from build123d import *

# Parameters (mm, degrees)
F0_R     = 10.16
F1_DEPTH = 15.7734
F3_DEPTH = 40.2336
F4_R     = 3.302


with BuildPart() as f1:
    # F0 (on Top) → F1 (new body)
    with BuildSketch(Plane.XY):
        with BuildLine():
            ThreePointArc((8.651677, 27.233786), (23.06244, 16.871706), (28.575, 0))
            ThreePointArc((28.575, 0), (22.710053, -17.343129), (7.522744, -27.56699))
            Line((7.522744, -27.56699), (57.294815, -18.7585))
            ThreePointArc((57.294815, -18.7585), (34.935126, -0.621041), (56.065332, 18.934968))
            Line((56.065332, 18.934968), (8.651677, 27.233786))
        make_face()
        with BuildLine():
            Line((58.440289, 18.519279), (56.065332, 18.934968))
            ThreePointArc((56.065332, 18.934968), (34.935126, -0.621041), (57.294815, -18.7585))
            ThreePointArc((57.294815, -18.7585), (68.572003, -12.240507), (73.025, 0))
            ThreePointArc((73.025, 0), (68.941066, 11.786406), (58.440289, 18.519279))
        make_face()
        with Locations((53.975, 0)):
            Circle(F0_R, mode=Mode.SUBTRACT)
    extrude(amount=F1_DEPTH)

    # F2 (on Top) → F3 (join)
    with BuildSketch(Plane.XY):
        with BuildLine():
            ThreePointArc((7.522744, -27.56699), (22.710053, -17.343129), (28.575, 0))
            ThreePointArc((28.575, 0), (23.06244, 16.871706), (8.651677, 27.233786))
            ThreePointArc((8.651677, 27.233786), (-28.568938, 0.58854), (7.522744, -27.56699))
        make_face()
        with BuildLine():
            ThreePointArc((13.447765, -4.826), (-14.2875, 0), (13.447765, 4.826))
            Line((13.447765, 4.826), (18.5293, 4.826))
            Line((18.5293, 4.826), (18.5293, -4.826))
            Line((18.5293, -4.826), (13.447765, -4.826))
        make_face(mode=Mode.SUBTRACT)
    extrude(amount=F3_DEPTH)

    # F4
    f4_edges = [f1.edges().sort_by_distance(p)[0] for p in [
        (-7.522744, 27.56699, 40.2336),
    ]]
    fillet(f4_edges, radius=F4_R)


solid = f1.part
CAD build for the part. Positions are in the model's coordinates, mm. A direction names the side the tool comes from. Round coordinates to 2 decimals unless told otherwise and drop trailing zeros. Write each loop counter-clockwise with the first axis right and the second up, starting at its lowest first coordinate (ties: lowest second). Pieces come first, ordered by that corner, then holes. Notation, with made-up numbers: M -29,50.5 L -21,50.5 A11 cw -21,62.5 Z; hole C -23.5,46.25 d8. An arc over 180 degrees is marked long. Use a Markdown table: item, result. Add a question column.
1. Slice it at C-C on x = 51.5. Give the cut face in (y, z), then the cut area to 3 significant figures.
2. Pull direction X, two halves, no side cores. Call faces 3 (the face through (11, -11, 40.234)), 4 (the face through (32.06, -23.224, 7.776)), 5 (the face through (18.529, 0, 20)): released by +X, released by -X, zero draft, split by the parting line, or undercut.
3. Flat gauge pins, fed straight in: P1, Ø1, axis at y = -18.5, z = 24, coming from the +X side; P2, Ø5.5, axis at x = 16, z = 16.5, coming from the +Y side; P3, Ø12, axis at x = 26.5, y = -20.5, coming from the +Z side. Where does each tip first touch, or does it go through?
4. Drill centre lines: probe 1 along Y at (x, z) = (-0.5, 12); probe 2 along X at (y, z) = (0, 28) (1 decimal); probe 3 along Z at (x, y) = (42.5, -2). Where is each one in solid material? Low to high.
5. Slice it at A-A on z = 9.5. Give the number of separate pieces and of enclosed holes in the cut face, then the cut area to 3 significant figures.
6. 3-axis set-ups, long thin cutter, end or side, ignore diameter. For faces 1 (the face through (22, 0, 0)), 2 (the face through (16, 4.826, 20)): which of +Z, -Z, +X, -X, +Y, -Y reach the whole face in a straight line?
Reply:
| question | item | result |
|---|---|---|
| 1 | outline | M -19.78,0 L -9.85,0 L -9.85,15.77 L -19.78,15.77 Z; M 9.85,0 L 19.73,0 L 19.73,15.77 L 9.85,15.77 Z |
| 1 | area | 312 mm^2 |
| 2 | face 3 | zero draft |
| 2 | face 4 | released by +X |
| 2 | face 5 | undercut |
| 3 | P1 | stops at x = 22.19 |
| 3 | P2 | stops at y = 26.41 |
| 3 | P3 | stops at z = 39.37 |
| 4 | probe 1 | y = -28.57 to -14.28, 14.28 to 28.57 |
| 4 | probe 2 | x = -28.6 to -14.3, 18.5 to 28.6 |
| 4 | probe 3 | z = 0 to 15.77 |
| 5 | separate pieces | 1 |
| 5 | enclosed holes | 2 |
| 5 | area | 3,440 mm^2 |
| 6 | face 1 | -Z, +X, -X, +Y, -Y |
| 6 | face 2 | +Z, -Z |
